Geometry: final body of the model. Coordinates: model frame, mm. A direction names the side the tool comes from. Round coordinates to 2 decimals unless told otherwise and drop trailing zeros. Loops run counter-clockwise (first coordinate to the right, second up) from the corner with the lowest first, then second, coordinate; pieces in that order, holes last. Notation, with made-up numbers: (69, 73.25) - (91, 73.25) arc R35 ccw to (91, 108.25) - close; hole circle Ø1 at (33, 39). An arc over 180 degrees is marked (long way). Answer as a JSON object with one key per item and string values. Group by question number.
Item 1: Section A-A (y = -44). Return the cut outline in (x, z), plus the area to 3 significant figures.
Item 2: Section C-C (z = 0). Return the cut outline in (x, y), plus the area to 3 significant figures.
Item 3: Section D-D (y = 0). Return the cut outline in (x, z), plus the area to 3 significant figures.
Item 4: Reachability of faces 1 (the face through (2, -15, 5.5)), 2 (the face through (2, -30.1, 0)), 3 (the face through (2, -25, -8)), 4 (the face through (4, -26, 0)), 5 (the face through (2, -58, 0)) from +Z, -Z, +X, -X, +Y, -Y: full face, straight path, thin tool, end or side. Return the list, or none.
Item 5: Line query: line 1 (Z direction, x = 2.8, y = -46.5); line 2 (Z direction, x = 2.7, y = 0); line 3 (Y direction, x = 2, z = -1.25). Output: solid intervals per line, ascending.
Item 6: First-contact query: pin 1 (1 mm diameter, centred on x = 1, z = -3, fed in from +Y); pin 2 (1.2 mm diameter, centred on x = 2.5, z = 9, fed in from +Y); pin 3 (1 mm diameter, centred on x = 3, y = -13.5, fed in from +Z); pin 4 (2 mm diameter, centred on y = -17, z = 8, fed in from -X). Flat tips, straight axial feed; report the tip coordinate or a pass-through.
Item 7: Draft query along Z for faces 6 (the face through (2, -42, -6.3)), 7 (the face through (2, 7, 0)), 8 (the face through (1.972, -56.498, -0.415)), 9 (the face through (2, -41, 10)). Return one class per face: released by +Z, released by -Z, zero draft, split by the parting line, or undercut.
Item 8: Section B-B (x = 3.05). Return the cut outline in (y, z), plus the area to 3 significant figures.
```python
from build123d import *

# Parameters (mm, degrees)
SKETCH1_R           = 7
BOSS_EXTRUDE1_DEPTH = 4
BOSS_EXTRUDE2_START = -5.5
SKETCH2_W           = 4
SKETCH2_H           = 36
BOSS_EXTRUDE2_DEPTH = 11
BOSS_EXTRUDE3_START = -10
SKETCH3_W           = 4
SKETCH3_H           = 33
BOSS_EXTRUDE3_DEPTH = 20
BOSS_EXTRUDE4_START = -1
SKETCH4_R           = 3.6
BOSS_EXTRUDE4_DEPTH = 6
BOSS_EXTRUDE5_START = -1
SKETCH5_R           = 0.9
BOSS_EXTRUDE5_DEPTH = 6
BOSS_EXTRUDE6_START = -1
SKETCH6_R           = 0.9
BOSS_EXTRUDE6_DEPTH = 6
BOSS_EXTRUDE7_START = -6.3
SKETCH7_W           = 6
SKETCH7_H           = 23.2
BOSS_EXTRUDE7_DEPTH = 12.6
BOSS_EXTRUDE8_START = -1
SKETCH8_R           = 0.9
BOSS_EXTRUDE8_DEPTH = 6
BOSS_EXTRUDE9_START = -1
SKETCH9_R           = 0.9
BOSS_EXTRUDE9_DEPTH = 6


with BuildPart() as part:
    # Sketch1 → Boss-Extrude1 (new body)
    with BuildSketch(Plane(origin=(0, 0, 0), x_dir=(0, 0, -1), z_dir=(1, 0, 0))):
        Circle(SKETCH1_R)
    extrude(amount=BOSS_EXTRUDE1_DEPTH)

    # Sketch2 → Boss-Extrude2 (add)
    with BuildSketch(Plane.XY.offset(BOSS_EXTRUDE2_START)):
        with Locations((2, -18)):
            Rectangle(SKETCH2_W, SKETCH2_H)
    extrude(amount=BOSS_EXTRUDE2_DEPTH)

    # Sketch3 → Boss-Extrude3 (add)
    with BuildSketch(Plane.XY.offset(BOSS_EXTRUDE3_START)):
        with Locations((2, -41.5)):
            Rectangle(SKETCH3_W, SKETCH3_H)
    extrude(amount=BOSS_EXTRUDE3_DEPTH)


with BuildPart() as body_2:
    # Sketch4 → Boss-Extrude4 (new body)
    with BuildSketch(Plane(origin=(0, 0, 0), x_dir=(0, 0, -1), z_dir=(1, 0, 0)).offset(BOSS_EXTRUDE4_START)):
        Circle(SKETCH4_R)
    extrude(amount=BOSS_EXTRUDE4_DEPTH)


with BuildPart() as part_1:
    add(part.part)

    # Combine1: cut body 2
    add(body_2.part, mode=Mode.SUBTRACT)


with BuildPart() as body_2_2:
    # Sketch5 → Boss-Extrude5 (new body)
    with BuildSketch(Plane(origin=(0, 0, 0), x_dir=(0, 0, -1), z_dir=(1, 0, 0)).offset(BOSS_EXTRUDE5_START)):
        with Locations((0, -7)):
            Circle(SKETCH5_R)
    extrude(amount=BOSS_EXTRUDE5_DEPTH)


with BuildPart() as part_2:
    add(part_1.part)

    # Combine2: cut body 2 2
    add(body_2_2.part, mode=Mode.SUBTRACT)


with BuildPart() as body_2_3:
    # Sketch6 → Boss-Extrude6 (new body)
    with BuildSketch(Plane(origin=(0, 0, 0), x_dir=(0, 0, -1), z_dir=(1, 0, 0)).offset(BOSS_EXTRUDE6_START)):
        with Locations((0, -14)):
            Circle(SKETCH6_R)
    extrude(amount=BOSS_EXTRUDE6_DEPTH)


with BuildPart() as part_3:
    add(part_2.part)

    # Combine3: cut body 2 3
    add(body_2_3.part, mode=Mode.SUBTRACT)


with BuildPart() as body_2_4:
    # Sketch7 → Boss-Extrude7 (new body)
    with BuildSketch(Plane.XY.offset(BOSS_EXTRUDE7_START)):
        with Locations((2, -41.7)):
            Rectangle(SKETCH7_W, SKETCH7_H)
    extrude(amount=BOSS_EXTRUDE7_DEPTH)


with BuildPart() as part_4:
    add(part_3.part)

    # Combine4: cut body 2 4
    add(body_2_4.part, mode=Mode.SUBTRACT)


with BuildPart() as body_2_5:
    # Sketch8 → Boss-Extrude8 (new body)
    with BuildSketch(Plane(origin=(0, 0, 0), x_dir=(0, 0, -1), z_dir=(1, 0, 0)).offset(BOSS_EXTRUDE8_START)):
        with Locations((0, -27.7)):
            Circle(SKETCH8_R)
    extrude(amount=BOSS_EXTRUDE8_DEPTH)


with BuildPart() as part_5:
    add(part_4.part)

    # Combine5: cut body 2 5
    add(body_2_5.part, mode=Mode.SUBTRACT)


with BuildPart() as body_2_6:
    # Sketch9 → Boss-Extrude9 (new body)
    with BuildSketch(Plane(origin=(0, 0, 0), x_dir=(0, 0, -1), z_dir=(1, 0, 0)).offset(BOSS_EXTRUDE9_START)):
        with Locations((0, -55.7)):
            Circle(SKETCH9_R)
    extrude(amount=BOSS_EXTRUDE9_DEPTH)


with BuildPart() as part_6:
    add(part_5.part)

    # Combine6: cut body 2 6
    add(body_2_6.part, mode=Mode.SUBTRACT)


solid = part_6.part
```
Values:
{
 "1": {"outline": "(0, -10) - (4, -10) - (4, -6.3) - (0, -6.3) - close; (0, 6.3) - (4, 6.3) - (4, 10) - (0, 10) - close", "area": "29.6 mm^2"},
 "2": {"outline": "(0, -58) - (4, -58) - (4, -56.6) - (0, -56.6) - close; (0, -54.8) - (4, -54.8) - (4, -53.3) - (0, -53.3) - close; (0, -30.1) - (4, -30.1) - (4, -28.6) - (0, -28.6) - close; (0, -26.8) - (4, -26.8) - (4, -14.9) - (0, -14.9) - close; (0, -13.1) - (4, -13.1) - (4, -7.9) - (0, -7.9) - close; (0, -6.1) - (4, -6.1) - (4, -3.6) - (0, -3.6) - close; (0, 3.6) - (4, 3.6) - (4, 7) - (0, 7) - close", "area": "110 mm^2"},
 "3": {"outline": "(0, -7) - (4, -7) - (4, -3.6) - (0, -3.6) - close; (0, 3.6) - (4, 3.6) - (4, 7) - (0, 7) - close", "area": "27.2 mm^2"},
 "4": {"face 1": "+Z, +X, -X", "face 2": "+X, -X", "face 3": "-Z, +X, -X", "face 4": "+Z, -Z, +X, +Y, -Y", "face 5": "+Z, -Z, +X, -X, -Y"},
 "5": {"line 1": "z = -10 to -6.3, 6.3 to 10", "line 2": "z = -7 to -3.6, 3.6 to 7", "line 3": "y = -58 to -53.3, -30.1 to -3.38, 3.38 to 6.89"},
 "6": {"pin 1": "stops at y = 6.54", "pin 2": "stops at y = -25", "pin 3": "stops at z = 5.5", "pin 4": "passes through"},
 "7": {"face 6": "undercut", "face 7": "split by the parting line", "face 8": "undercut", "face 9": "released by +Z"},
 "8": {"outline": "(-58, -10) - (-25, -10) - (-25, -5.5) - (-4.33, -5.5) arc R7 ccw (long way) to (-4.33, 5.5) - (-25, 5.5) - (-25, 10) - (-58, 10) - close; hole circle Ø1.8 at (-55.7, 0); hole (-53.3, -6.3) - (-30.1, -6.3) - (-30.1, 6.3) - (-53.3, 6.3) - close; hole circle Ø1.8 at (-27.7, 0); hole circle Ø1.8 at (-14, 0); hole circle Ø1.8 at (-7, 0); hole circle Ø7.2 at (0, 0)", "area": "678 mm^2"}
}
